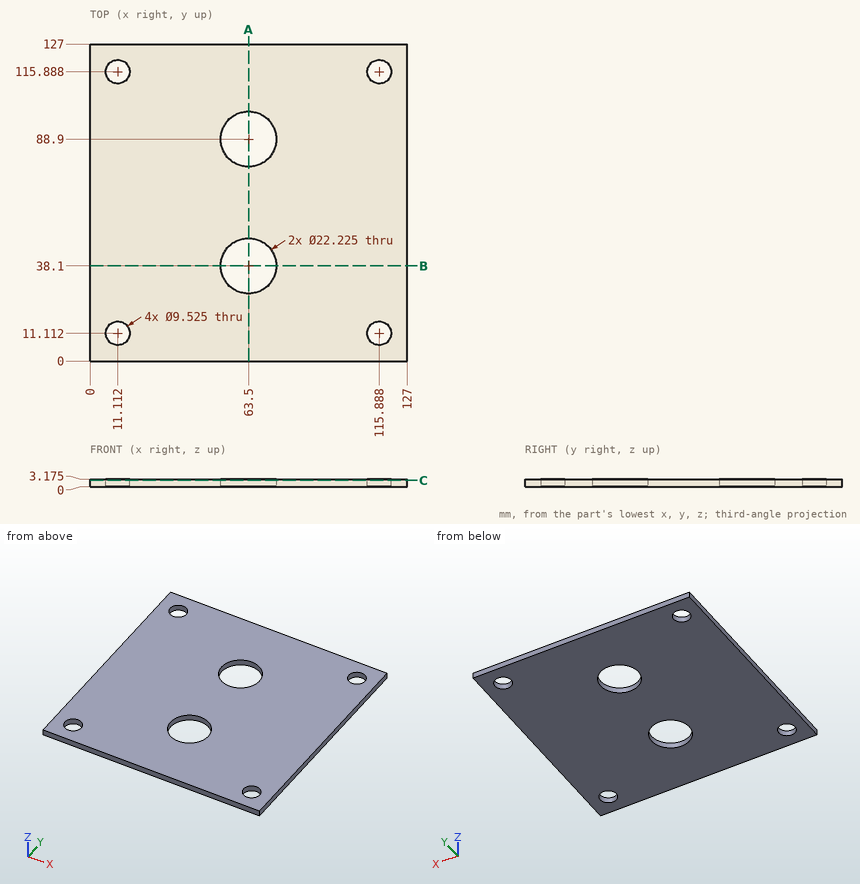
Print and shaded views of the part. All mm, measured from the part's lowest x, y and z. Coordinates: 2 decimals unless noted, no trailing zeros. Loops run counter-clockwise (first coordinate to the right, second up) from the corner with the lowest first, then second, coordinate; pieces in that order, holes last. Notation, with made-up numbers: (69, -26.5) -> (83, -26.5) arc R14 ccw to (83, -12.5) -> close; hole circle Ø10 at (-22, 52.5). An arc over 180 degrees is marked (long way). Use a Markdown table: item, result. Add a question column.
Item 1: Probe probe 1 along Y at (x, z) = (11, 1.45); probe 2 along Y at (x, z) = (63.5, 1.1); probe 3 along X at (y, z) = (15, 0.4) (1 decimal). List the from-to ranges inside material, lowest first.
Item 2: Band-saw the part on B-B on y = 38.1. Write the cut outline in (x, z) (1 decimal).
Item 3: Band-saw the part on C-C on z = 2.65. Give the number of separate pieces and of enclosed holes in the cut face, plus the area to 3 significant figures.
Item 4: Band-saw the part on A-A on x = 63.5. Write the cut outline in (y, z) (1 decimal), plus the area to 3 significant figures.
Geometry says:
| question | item | result |
|---|---|---|
| 1 | probe 1 | 0 to 6.35, 15.87 to 111.13, 120.65 to 127 |
| 1 | probe 2 | 0 to 26.99, 49.21 to 77.79, 100.01 to 127 |
| 1 | probe 3 | 0 to 8.4, 13.9 to 113.1, 118.6 to 127 |
| 2 | outline | (0, 0) -> (52.4, 0) -> (52.4, 3.2) -> (0, 3.2) -> close; (74.6, 0) -> (127, 0) -> (127, 3.2) -> (74.6, 3.2) -> close |
| 3 | separate pieces | 1 |
| 3 | enclosed holes | 6 |
| 3 | area | 15,100 mm² |
| 4 | outline | (0, 0) -> (27, 0) -> (27, 3.2) -> (0, 3.2) -> close; (49.2, 0) -> (77.8, 0) -> (77.8, 3.2) -> (49.2, 3.2) -> close; (100, 0) -> (127, 0) -> (127, 3.2) -> (100, 3.2) -> close |
| 4 | area | 262 mm² |
